Input: dimensioned drawing with shaded views. Units: mm. Origin: part minimum x, y, z. Give positions to 0.01 mm unless a question says otherwise; leave off trailing zeros. Loops run counter-clockwise (first coordinate to the right, second up) from the corner with the lowest first, then second, coordinate; pieces in that order, holes last. Notation, with made-up numbers: M 62.5,76.5 L 110.5,76.5 A18 cw 110.5,99.5 Z; hole C -36.5,38.5 d2. An arc over 180 degrees is marked long. Answer in a Markdown table with one row per item.
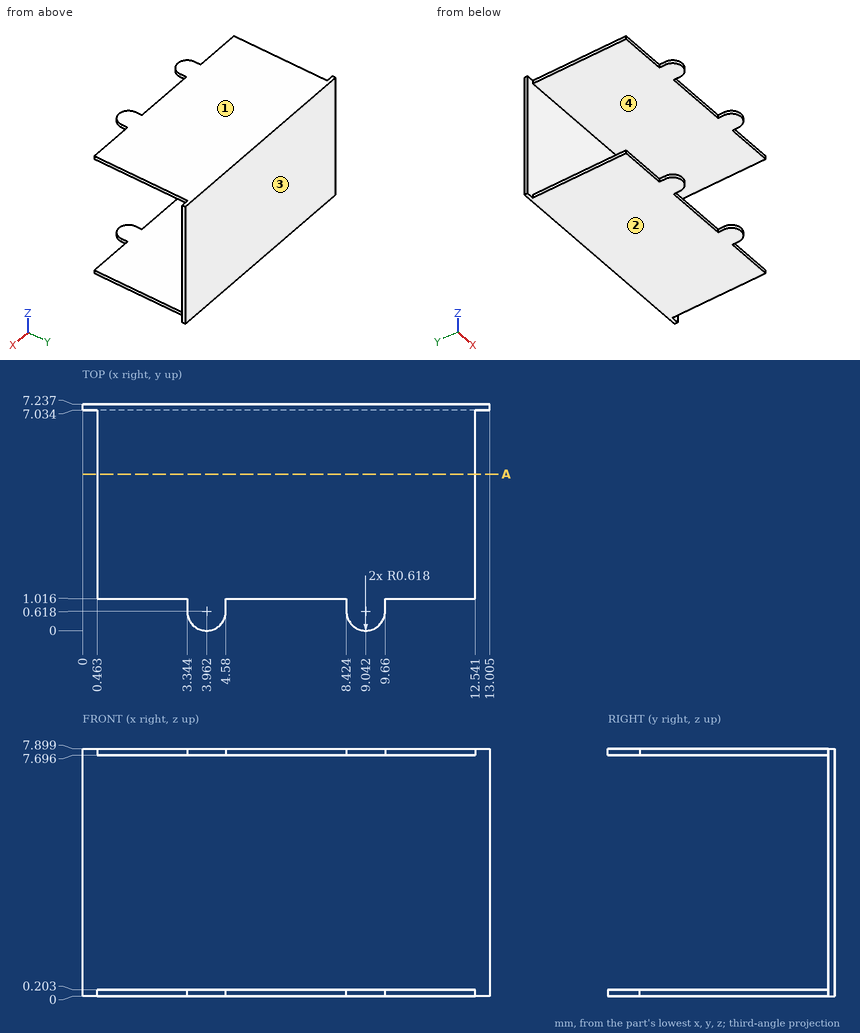
Q1. Ray query, probe 1 along Z at (x, y) = (1, 5.75); probe 2 along Y at (x, z) = (3.75, 4.75) (1 decimal); probe 3 along X at (y, z) = (1.25, 7.75). Return the intervals inside material, ascending. Write a range as from..to.
Values follow:
| item | result |
|---|---|
| probe 1 | 0..0.2, 7.7..7.9 |
| probe 2 | 7..7.2 |
| probe 3 | 0.46..12.54 |
Q2. Section query A-A (y = 5). Output: boundary loops of the cut face in (x, z).
Values follow:
| item | result |
|---|---|
| outline | M 0.46,0 L 12.54,0 L 12.54,0.2 L 0.46,0.2 Z; M 0.46,7.7 L 12.54,7.7 L 12.54,7.9 L 0.46,7.9 Z |
Q3. Mould query, pull axis Z, two halves, no side actions, for the marked faces 1, 2, 3 and 4. Classes: +Z half, -Z half, draft (parallel to the pull), parting line (faces both ways), or undercut.
Values follow:
| item | result |
|---|---|
| face 1 | +Z half |
| face 2 | -Z half |
| face 3 | draft |
| face 4 | undercut |
Q4. Contact query for a flat-ended pin moving along its axis: pin 1 Ø4 at (y, z) = (3, 1.5) entering from +X. Output: stop coordinate, or through.
Values follow:
| item | result |
|---|---|
| pin 1 | x = 12.54 |
